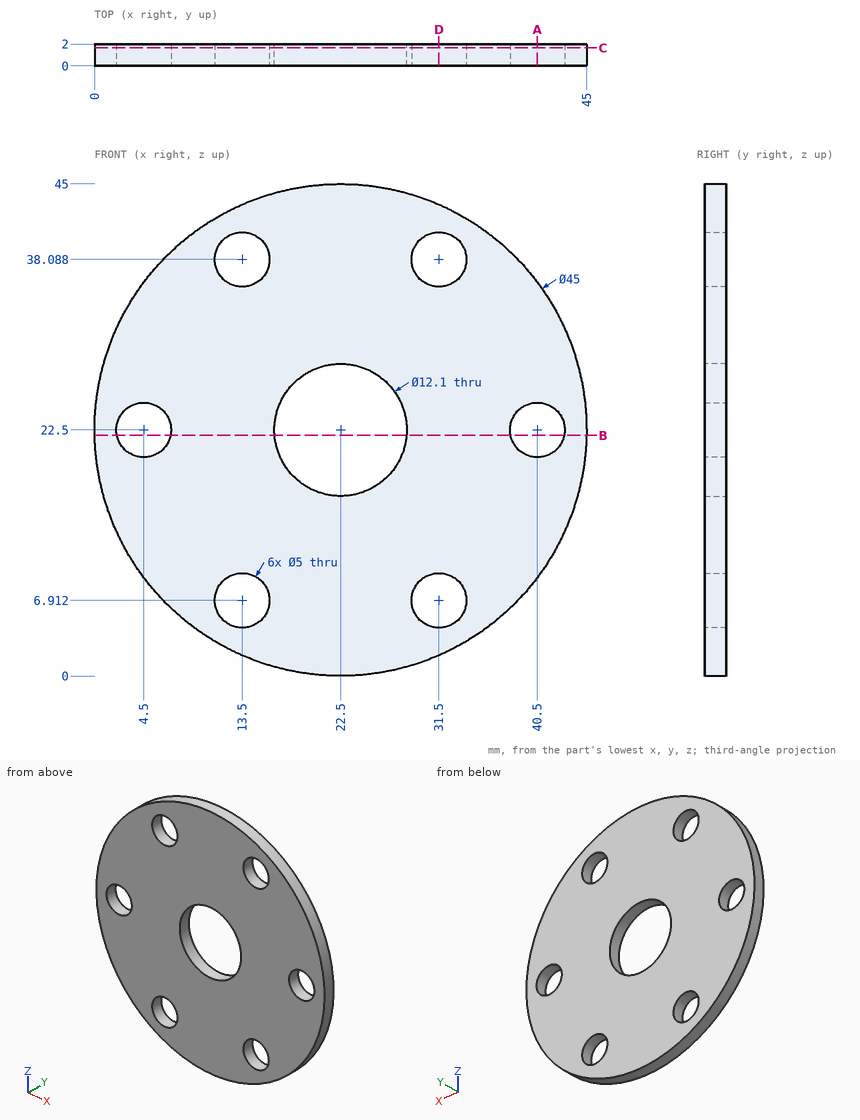
Study the drawing (mm; zero at the part's minimum x, y, z) and answer. Give positions to 0.01 mm unless a question says otherwise; leave off trailing zeros. Write each loop counter-clockwise with the first axis right and the second up, starting at its lowest first coordinate (ties: lowest second). Pieces come first, ordered by that corner, then holes.
Item 1: Section D-D, the plane x = 31.5 is taken. Write down the section's boundary in (y, z).
Item 2: Section B-B, the plane z = 22 is taken. Count the separate pieces of the cut face and the enclosed holes in it.
Item 3: Section C-C, the plane y = 1.65 is taken. Write down the section's boundary in (x, z), plus the area to 3 significant figures.
Item 4: Find the intervals of material crossed by line 1 along Z through (x, y) = (13, 1.4) (1 decimal); line 2 along X through (y, z) = (0.95, 22.5); line 3 along X through (y, z) = (1.85, 21.5), in increasing order.
Item 5: Section A-A, the plane x = 40.5 is taken. Write down the section's boundary in (y, z), plus the area to 3 significant figures.
Completed:
1. outline: (0, 1.88) - (2, 1.88) - (2, 4.41) - (0, 4.41) - close; (0, 9.41) - (2, 9.41) - (2, 35.59) - (0, 35.59) - close; (0, 40.59) - (2, 40.59) - (2, 43.12) - (0, 43.12) - close
2. separate pieces: 4
2. enclosed holes: 0
3. outline: circle Ø45 at (22.5, 22.5); hole circle Ø5 at (4.5, 22.5); hole circle Ø5 at (13.5, 6.91); hole circle Ø5 at (13.5, 38.09); hole circle Ø12.1 at (22.5, 22.5); hole circle Ø5 at (31.5, 6.91); hole circle Ø5 at (31.5, 38.09); hole circle Ø5 at (40.5, 22.5)
3. area: 1,360 mm2
4. line 1: z = 2.1 to 4.5, 9.4 to 35.6, 40.5 to 42.9
4. line 2: x = 0 to 2, 7 to 16.45, 28.55 to 38, 43 to 45
4. line 3: x = 0.02 to 2.21, 6.79 to 16.53, 28.47 to 38.21, 42.79 to 44.98
5. outline: (0, 9) - (2, 9) - (2, 20) - (0, 20) - close; (0, 25) - (2, 25) - (2, 36) - (0, 36) - close
5. area: 44.0 mm2
